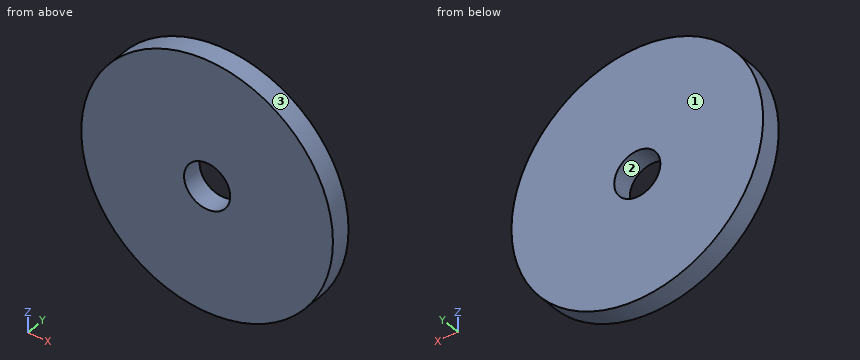
from build123d import *

# Parameters (mm, degrees)
CYLINDER011007_R     = 2.2
CYLINDER011007_DEPTH = 20
CYLINDER011008_R     = 12
CYLINDER011008_DEPTH = 2


with BuildPart() as belt_attach_insert_hole:
    # Cylinder011007 → Cylinder011007 (new body)
    with BuildSketch(Plane.XZ):
        Circle(CYLINDER011007_R)
    extrude(amount=CYLINDER011007_DEPTH)


with BuildPart() as obj1:
    # Cylinder011008 → Cylinder011008 (new body)
    with BuildSketch(Plane.XZ):
        Circle(CYLINDER011008_R)
    extrude(amount=CYLINDER011008_DEPTH)

    # Cut023015009008: cut belt attach insert hole
    add(belt_attach_insert_hole.part, mode=Mode.SUBTRACT)


solid = obj1.part
Read the model definition and answer for the solid it produces. Units are mm, in the model's axes. Face numbers are marked on the shaded views. Give positions to 0.01 mm unless a question says otherwise; leave off trailing zeros. Write each loop counter-clockwise with the first axis right and the second up, starting at its lowest first coordinate (ties: lowest second). Pieces come first, ordered by that corner, then holes. Notation, with made-up numbers: M 49.25,49.25 L 105.25,49.25 A11 cw 105.25,55.25 Z; hole C 86,-1 d7. An arc over 180 degrees is marked long. One line per item, written item: value. Start each with the question number.
(1) Find section C-C (y = -1.2). Determine the outline of the cut face in (x, z).
(2) A flat-ended cylindrical pin translates along its axis: pin 1 Ø1 at (y, z) = (-0.5, -1) entering from +X. Find the tip coordinate at first contact, or state that the pin passes through.
(3) Find section D-D (x = 6.25). Determine the outline of the cut face in (y, z), plus the area to 3 significant figures.
(4) Find section B-B (x = 0). Determine the outline of the cut face in (y, z), plus the area to 3 significant figures.
(5) Determine the mould class of the marked faces 1, 2 and 3 for opening direction X: pulls with the +X half, pulls with the -X half, needs draft (parallel to the pull), parting line crosses it, or undercut.
(6) Find section A-A (z = 0). Determine the outline of the cut face in (x, y), plus the area to 3 significant figures.
(7) Find the intervals of material crossed by line 1 (Z direction, x = 0, y = -1.55); line 2 (Z direction, x = -1, y = -1.55); line 3 (X direction, y = -0.6, z = 2), in increasing order.
Results below:
1. outline: C 0,0 d24; hole C 0,0 d4.4
2. pin 1: stops at x = 11.99
3. outline: M -2,-10.24 L 0,-10.24 L 0,10.24 L -2,10.24 Z
3. area: 41.0 mm^2
4. outline: M -2,-12 L 0,-12 L 0,-2.2 L -2,-2.2 Z; M -2,2.2 L 0,2.2 L 0,12 L -2,12 Z
4. area: 39.2 mm^2
5. face 1: needs draft
5. face 2: undercut
5. face 3: parting line crosses it
6. outline: M -12,-2 L -2.2,-2 L -2.2,0 L -12,0 Z; M 2.2,-2 L 12,-2 L 12,0 L 2.2,0 Z
6. area: 39.2 mm^2
7. line 1: z = -12 to -2.2, 2.2 to 12
7. line 2: z = -11.96 to -1.96, 1.96 to 11.96
7. line 3: x = -11.83 to -0.92, 0.92 to 11.83
